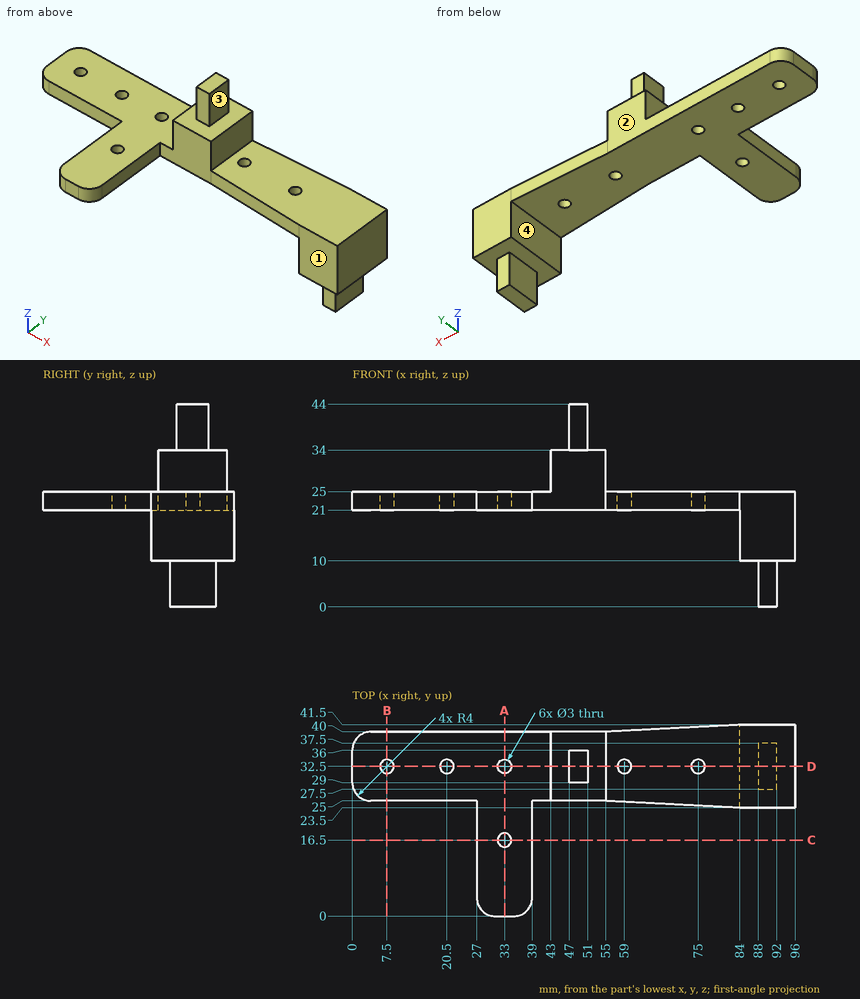
Answer from the drawing. Dimensions are ordinates in mm from the lowest x, y and z of the part. A direction names the side the tool comes from. Coordinates: 2 decimals unless noted, no trailing zeros. Order: outer loops, then holes, each group sorted by start corner. A loop starts at its lowest first (then second) coordinate and runs counter-clockwise, first axis right, second up. Notation, with made-up numbers: (84, 65.25) -> (92, 65.25) arc R26 ccw to (92, 88.25) -> close; hole circle Ø10 at (64, 23). An arc over 180 degrees is marked (long way). Answer as a JSON object with one key per item and string values.
1) A cutting plane is placed at B-B, the plane x = 7.5. Determine the outline of the cut face in (y, z), plus the area to 3 significant figures.
Model answer:
{"outline": "(25, 21) -> (31, 21) -> (31, 25) -> (25, 25) -> close; (34, 21) -> (40, 21) -> (40, 25) -> (34, 25) -> close", "area": "48.0 mm²"}
2) Each of these flat-tipped pins is pushed along its axis until it touches: pin 1 (12 mm diameter, centred on y = 34, z = 14, fed in from -X); pin 2 (4.5 mm diameter, centred on y = 12.5, z = 23, fed in from -X); pin 3 (8 mm diameter, centred on x = 32.5, y = 8.5, fed in from -Z). Where does it stop, or does it pass through?
Model answer:
{"pin 1": "stops at x = 84", "pin 2": "stops at x = 27", "pin 3": "stops at z = 21"}
3) A tool of negligible diameter and unlimited length cuts with its end or side. For the marked faces 1, 2, 3 and 4, from which of +Z, -Z, +X, -X, +Y, -Y can it reach the whole face along a straight path? Write none if from no direction.
Model answer:
{"face 1": "+Z, -Z, +X, -Y", "face 2": "+Z, -Z, -X, +Y", "face 3": "+Z, +X, +Y, -Y", "face 4": "-Z, -X, +Y, -Y"}
4) Consider line 1 along Y through (x, z) = (33, 23); line 2 along X through (y, z) = (34.5, 20); line 3 along X through (y, z) = (12, 22). Determine where each line is inside the solid, lowest interval first. Write a range as from..to.
Model answer:
{"line 1": "y = 0..15, 18..31, 34..40", "line 2": "x = 84..96", "line 3": "x = 27..39"}
5) A cutting plane is placed at D-D, the plane y = 32.5. State how many separate pieces and enclosed holes the cut face has, plus the area to 3 significant figures.
Model answer:
{"separate pieces": "6", "enclosed holes": "0", "area": "644 mm²"}
6) A cutting plane is placed at A-A, the plane x = 33. Determine the outline of the cut face in (y, z), plus the area to 3 significant figures.
Model answer:
{"outline": "(0, 21) -> (15, 21) -> (15, 25) -> (0, 25) -> close; (18, 21) -> (31, 21) -> (31, 25) -> (18, 25) -> close; (34, 21) -> (40, 21) -> (40, 25) -> (34, 25) -> close", "area": "136 mm²"}
7) A cutting plane is placed at C-C, the plane y = 16.5. Determine the outline of the cut face in (x, z).
Model answer:
{"outline": "(27, 21) -> (31.5, 21) -> (31.5, 25) -> (27, 25) -> close; (34.5, 21) -> (39, 21) -> (39, 25) -> (34.5, 25) -> close"}
